from build123d import *

# Parameters (mm, degrees)
SALIENTE_EXTRUIR1_DEPTH = 16
CORTAR_EXTRUIR1_REACH   = 45.239
CROQUIS2_W              = 5.2
CROQUIS2_H              = 2.75
CROQUIS2_R              = 2.5
CROQUIS5_W              = 4
CROQUIS5_H              = 2.2
SALIENTE_EXTRUIR4_DEPTH = 12.2
CROQUIS6_W              = 8
CROQUIS6_H              = 2.2
SALIENTE_EXTRUIR5_DEPTH = 9
REDONDEO2_R             = 2.7


with BuildPart() as part:
    # Croquis1 → Saliente-Extruir1 (new body)
    with BuildSketch(Plane.XY):
        with BuildLine():
            Line((0, -8.2), (38.8, -8.2))
            Line((38.8, -8.2), (38.8, -10.4))
            Line((38.8, -10.4), (0, -10.4))
            ThreePointArc((0, -10.4), (-5.2, -5.2), (0, 0))
            Line((0, 0), (38.8, 0))
            Line((38.8, 0), (38.8, -2.2))
            Line((38.8, -2.2), (0, -2.2))
            ThreePointArc((0, -2.2), (-3, -5.2), (0, -8.2))
        make_face()
    extrude(amount=SALIENTE_EXTRUIR1_DEPTH)

    # Cortar-Extruir1: up to this face of the body (flat: up to its plane)
    cortar_extruir1_end = Plane(part.part.faces().sort_by_distance((19.4, -10.4, 8))[0])
    # Croquis2 → Cortar-Extruir1 (cut, up to the picked face)
    with BuildSketch(Plane(origin=(0, 0, 0), x_dir=(1, 0, 0), z_dir=(0, 1, 0)), mode=Mode.PRIVATE) as cortar_extruir1_sk1:
        with Locations((-2.6, -8)):
            Rectangle(CROQUIS2_W, CROQUIS2_H)
    cortar_extruir1_tool1 = split(extrude(cortar_extruir1_sk1.sketch, amount=-CORTAR_EXTRUIR1_REACH, mode=Mode.PRIVATE), bisect_by=cortar_extruir1_end, keep=Keep.BOTH, mode=Mode.PRIVATE)
    # Croquis2 → Cortar-Extruir1 (cut, up to the picked face)
    with BuildSketch(Plane(origin=(0, 0, 0), x_dir=(1, 0, 0), z_dir=(0, 1, 0)), mode=Mode.PRIVATE) as cortar_extruir1_sk2:
        with BuildLine():
            Line((4.36594372, -6.625), (0, -6.625))
            Line((0, -6.625), (0, -9.375))
            Line((0, -9.375), (4.36594372, -9.375))
            ThreePointArc((4.36594372, -9.375), (4.05, -8), (4.36594372, -6.625))
        make_face()
    cortar_extruir1_tool2 = split(extrude(cortar_extruir1_sk2.sketch, amount=-CORTAR_EXTRUIR1_REACH, mode=Mode.PRIVATE), bisect_by=cortar_extruir1_end, keep=Keep.BOTH, mode=Mode.PRIVATE)
    # Croquis2 → Cortar-Extruir1 (cut, up to the picked face)
    with BuildSketch(Plane(origin=(0, 0, 0), x_dir=(1, 0, 0), z_dir=(0, 1, 0)), mode=Mode.PRIVATE) as cortar_extruir1_sk3:
        with BuildLine():
            ThreePointArc((10.03405628, -6.625), (7.2, -4.85), (4.36594372, -6.625))
            Line((4.36594372, -6.625), (10.03405628, -6.625))
        make_face()
    cortar_extruir1_tool3 = split(extrude(cortar_extruir1_sk3.sketch, amount=-CORTAR_EXTRUIR1_REACH, mode=Mode.PRIVATE), bisect_by=cortar_extruir1_end, keep=Keep.BOTH, mode=Mode.PRIVATE)
    # Croquis2 → Cortar-Extruir1 (cut, up to the picked face)
    with BuildSketch(Plane(origin=(0, 0, 0), x_dir=(1, 0, 0), z_dir=(0, 1, 0)), mode=Mode.PRIVATE) as cortar_extruir1_sk4:
        with BuildLine():
            Line((10.03405628, -6.625), (4.36594372, -6.625))
            ThreePointArc((4.36594372, -6.625), (4.05, -8), (4.36594372, -9.375))
            Line((4.36594372, -9.375), (10.03405628, -9.375))
            ThreePointArc((10.03405628, -9.375), (10.26999815, -8.705415735), (10.35, -8))
            ThreePointArc((10.35, -8), (10.26999815, -7.294584265), (10.03405628, -6.625))
        make_face()
    cortar_extruir1_tool4 = split(extrude(cortar_extruir1_sk4.sketch, amount=-CORTAR_EXTRUIR1_REACH, mode=Mode.PRIVATE), bisect_by=cortar_extruir1_end, keep=Keep.BOTH, mode=Mode.PRIVATE)
    # Croquis2 → Cortar-Extruir1 (cut, up to the picked face)
    with BuildSketch(Plane(origin=(0, 0, 0), x_dir=(1, 0, 0), z_dir=(0, 1, 0)), mode=Mode.PRIVATE) as cortar_extruir1_sk5:
        with BuildLine():
            Line((10.03405628, -9.375), (4.36594372, -9.375))
            ThreePointArc((4.36594372, -9.375), (7.2, -11.15), (10.03405628, -9.375))
        make_face()
    cortar_extruir1_tool5 = split(extrude(cortar_extruir1_sk5.sketch, amount=-CORTAR_EXTRUIR1_REACH, mode=Mode.PRIVATE), bisect_by=cortar_extruir1_end, keep=Keep.BOTH, mode=Mode.PRIVATE)
    # Croquis2 → Cortar-Extruir1 (cut, up to the picked face)
    with BuildSketch(Plane(origin=(0, 0, 0), x_dir=(1, 0, 0), z_dir=(0, 1, 0)), mode=Mode.PRIVATE) as cortar_extruir1_sk6:
        with BuildLine():
            Line((11.925, -6.625), (10.03405628, -6.625))
            ThreePointArc((10.03405628, -6.625), (10.26999815, -7.294584265), (10.35, -8))
            ThreePointArc((10.35, -8), (10.26999815, -8.705415735), (10.03405628, -9.375))
            Line((10.03405628, -9.375), (11.925, -9.375))
            ThreePointArc((11.925, -9.375), (13.3, -8), (11.925, -6.625))
        make_face()
    cortar_extruir1_tool6 = split(extrude(cortar_extruir1_sk6.sketch, amount=-CORTAR_EXTRUIR1_REACH, mode=Mode.PRIVATE), bisect_by=cortar_extruir1_end, keep=Keep.BOTH, mode=Mode.PRIVATE)
    # Croquis2 → Cortar-Extruir1 (cut, up to the picked face)
    with BuildSketch(Plane(origin=(0, 0, 0), x_dir=(1, 0, 0), z_dir=(0, 1, 0)), mode=Mode.PRIVATE) as cortar_extruir1_sk7:
        with Locations(Location((30.8, -8, 0), (0, 0, 180))):
            Circle(CROQUIS2_R)
    cortar_extruir1_tool7 = split(extrude(cortar_extruir1_sk7.sketch, amount=-CORTAR_EXTRUIR1_REACH, mode=Mode.PRIVATE), bisect_by=cortar_extruir1_end, keep=Keep.BOTH, mode=Mode.PRIVATE)
    # Croquis2 → Cortar-Extruir1 (cut, up to the picked face)
    with BuildSketch(Plane(origin=(0, 0, 0), x_dir=(1, 0, 0), z_dir=(0, 1, 0)), mode=Mode.PRIVATE) as cortar_extruir1_sk8:
        with BuildLine():
            Line((38.8, 0), (30.8, 0))
            ThreePointArc((30.8, 0), (36.456854249, -2.343145751), (38.8, -8))
            Line((38.8, -8), (38.8, 0))
        make_face()
    cortar_extruir1_tool8 = split(extrude(cortar_extruir1_sk8.sketch, amount=-CORTAR_EXTRUIR1_REACH, mode=Mode.PRIVATE), bisect_by=cortar_extruir1_end, keep=Keep.BOTH, mode=Mode.PRIVATE)
    # Croquis2 → Cortar-Extruir1 (cut, up to the picked face)
    with BuildSketch(Plane(origin=(0, 0, 0), x_dir=(1, 0, 0), z_dir=(0, 1, 0)), mode=Mode.PRIVATE) as cortar_extruir1_sk9:
        with BuildLine():
            Line((38.8, -16), (38.8, -8))
            ThreePointArc((38.8, -8), (36.456854249, -13.656854249), (30.8, -16))
            Line((30.8, -16), (38.8, -16))
        make_face()
    cortar_extruir1_tool9 = split(extrude(cortar_extruir1_sk9.sketch, amount=-CORTAR_EXTRUIR1_REACH, mode=Mode.PRIVATE), bisect_by=cortar_extruir1_end, keep=Keep.BOTH, mode=Mode.PRIVATE)
    add(cortar_extruir1_tool1.solids().sort_by(Axis((-2.6, 0, 8), (0, -1, 0)))[0], mode=Mode.SUBTRACT)
    add(cortar_extruir1_tool2.solids().sort_by(Axis((2.077605, 0, 8), (0, -1, 0)))[0], mode=Mode.SUBTRACT)
    add(cortar_extruir1_tool3.solids().sort_by(Axis((7.2, 0, 5.894461), (0, -1, 0)))[0], mode=Mode.SUBTRACT)
    add(cortar_extruir1_tool4.solids().sort_by(Axis((7.2, 0, 8), (0, -1, 0)))[0], mode=Mode.SUBTRACT)
    add(cortar_extruir1_tool5.solids().sort_by(Axis((7.2, 0, 10.105539), (0, -1, 0)))[0], mode=Mode.SUBTRACT)
    add(cortar_extruir1_tool6.solids().sort_by(Axis((11.641399, 0, 8), (0, -1, 0)))[0], mode=Mode.SUBTRACT)
    add(cortar_extruir1_tool7.solids().sort_by(Axis((30.8, 0, 8), (0, -1, 0)))[0], mode=Mode.SUBTRACT)
    add(cortar_extruir1_tool8.solids().sort_by(Axis((37.013056, 0, 1.786944), (0, -1, 0)))[0], mode=Mode.SUBTRACT)
    add(cortar_extruir1_tool9.solids().sort_by(Axis((37.013056, 0, 14.213056), (0, -1, 0)))[0], mode=Mode.SUBTRACT)

    # Croquis5 → Saliente-Extruir4 (add)
    with BuildSketch(Plane.XY.offset(16)):
        with Locations((5.2, -9.3)):
            Rectangle(CROQUIS5_W, CROQUIS5_H)
        with Locations((9.2, -9.3)):
            Rectangle(CROQUIS5_W, CROQUIS5_H)
    extrude(amount=SALIENTE_EXTRUIR4_DEPTH)

    # Croquis6 → Saliente-Extruir5 (add)
    with BuildSketch(Plane(origin=(0, -8.2, 0), x_dir=(1, 0, 0), z_dir=(0, 1, 0))):
        with Locations((7.2, -27.1)):
            Rectangle(CROQUIS6_W, CROQUIS6_H)
    extrude(amount=SALIENTE_EXTRUIR5_DEPTH)

    # Redondeo2
    redondeo2_edges = [part.edges().sort_by_distance(p)[0] for p in [
        (7.2, -10.4, 28.2),
    ]]
    fillet(redondeo2_edges, radius=REDONDEO2_R)


solid = part.part
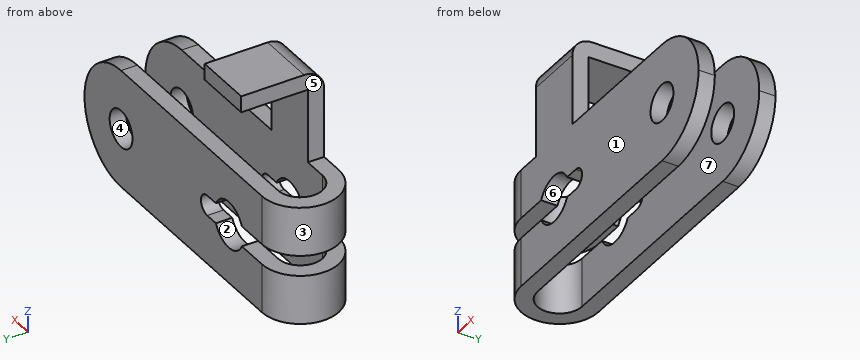
Source: CAD feature listing. Evaluate the final solid. Frame: model axes, mm. Face numbers are marked on the shaded views. A direction names the side the tool comes from. Round coordinates to 2 decimals unless told otherwise and drop trailing zeros. Loops run counter-clockwise (first coordinate to the right, second up) from the corner with the lowest first, then second, coordinate; pieces in that order, holes last. Notation, with made-up numbers: (-16, 32.25) -> (2, 32.25) arc R24 ccw to (2, 54.25) -> close; hole circle Ø4 at (-35, 52.25). An arc over 180 degrees is marked (long way). Answer as a JSON object with one key per item and string values. Group by question number.
Q1. Section query A-A (y = -5.2). Output: boundary loops of the cut face in (x, z) (3 decimals), plus the area to 4 significant figures.
Q2. Access query for the marked faces 5, 6 and 7. Directions: +Z, -Z, +X, -X, +Y, -Y. A direction counts if a zero-diameter tool reaches every point of the face in a straight line with its end or side. Return the directions, or none.
Q3. Ray query, line 1 (Y direction, x = 26, z = 7.5); line 2 (Z direction, x = 30.8, y = -1.55); line 3 (X direction, y = -9.25, z = 10). Return the intervals inside material, ascending. Write a range as from..to.
Q4. Section query B-B (x = 17). Output: boundary loops of the cut face in (y, z).
Q5. Contact query for flat-ended pins moving along their axis: P1, Ø5, axis at x = -2, y = -5, coming from the +Z side; P2, Ø10, axis at x = 14, z = 5.5, coming from the +Y side; P3, Ø1.5, axis at x = 11, y = -9.5, coming from the +Z side. Output: stop coordinate, or through.
Q6. Section query C-C (y = -1.25). Output: boundary loops of the cut face in (x, z) (3 decimals), plus the area to 3 significant figures.
Q7. Mould query, pull axis X, two halves, no side actions, for the marked faces 1, 2, 3 and 4. Classes: pulls with the +X half, pulls with the -X half, needs draft (parallel to the pull), parting line crosses it, or undercut.
Q8. Section query D-D (z = 6). Output: boundary loops of the cut face in (x, y), plus the area to 3 significant figures.
Completed:
{
 "1": {"outline": "(-5.2, 0) -> (-3, 0) -> (-3, 6.625) -> (-5.2, 6.625) -> close; (-5.2, 9.375) -> (-3, 9.375) -> (-3, 16) -> (-5.2, 16) -> close; (3.2, 26) -> (11.2, 26) -> (11.2, 28.2) -> (3.2, 28.2) -> close", "area": "46.75 mm²"},
 "2": {"face 5": "+Z, -X, +Y, -Y", "face 6": "+Y, -Y", "face 7": "-Z, +X"},
 "3": {"line 1": "-10.4..-8.2, -2.2..0", "line 2": "0..5.5, 10.5..16", "line 3": "-3.26..4.77, 9.63..29.3, 32.3..38.55"},
 "4": {"outline": "(-10.4, 0) -> (-8.2, 0) -> (-8.2, 16) -> (-10.4, 16) -> close; (-2.2, 0) -> (0, 0) -> (0, 16) -> (-2.2, 16) -> close"},
 "5": {"P1": "z = 16", "P2": "y = 0", "P3": "z = 27.99"},
 "6": {"outline": "(-3.382, 0) -> (30.8, 0) arc R8 ccw to (30.8, 16) -> (-3.382, 16) -> (-3.382, 9.375) -> (4.366, 9.375) arc R3.15 cw to (10.034, 9.375) -> (11.925, 9.375) arc R1.375 cw to (11.925, 6.625) -> (10.034, 6.625) arc R3.15 cw to (4.366, 6.625) -> (-3.382, 6.625) -> close; (3.2, 26) -> (11.2, 26) -> (11.2, 28.2) -> (3.2, 28.2) -> close; hole circle Ø5 at (30.8, 8)", "area": "586 mm²"},
 "7": {"face 1": "needs draft", "face 2": "undercut", "face 3": "pulls with the -X half", "face 4": "undercut"},
 "8": {"outline": "(0, -10.4) -> (4.77, -10.4) -> (4.77, -8.2) -> (0, -8.2) arc R3 cw to (0, -2.2) -> (4.77, -2.2) -> (4.77, 0) -> (0, 0) arc R5.2 ccw to start; (9.63, -10.4) -> (29.3, -10.4) -> (29.3, -8.2) -> (9.63, -8.2) -> close; (9.63, -2.2) -> (29.3, -2.2) -> (29.3, 0) -> (9.63, 0) -> close; (32.3, -10.4) -> (38.55, -10.4) -> (38.55, -8.2) -> (32.3, -8.2) -> close; (32.3, -2.2) -> (38.55, -2.2) -> (38.55, 0) -> (32.3, 0) -> close", "area": "163 mm²"}
}
